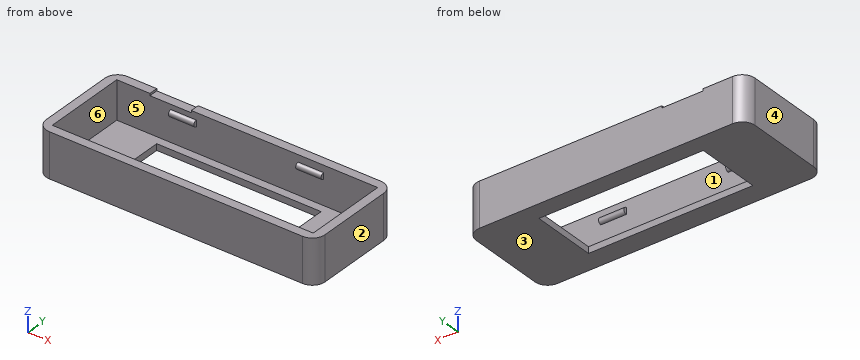
```python
from build123d import *

# Parameters (mm, degrees)
SKETCH010_W     = 43.8
SKETCH010_H     = 16.05
SKETCH010_W_2   = 41
SKETCH010_H_2   = 13.25
PAD004_DEPTH    = 6
SKETCH011_W     = 43.8
SKETCH011_H     = 16.05
SKETCH011_W_2   = 25.832
SKETCH011_H_2   = 10.205235
PAD005_DEPTH    = 1
FILLET_R        = 2
SKETCH012_W     = 6.5
SKETCH012_H     = 4.714983
POCKET004_DEPTH = 8.026
SKETCH027_R     = 0.5
PAD006_DEPTH    = 2


with BuildPart() as part:
    # Sketch010 → Pad004 (new body)
    with BuildSketch(Plane.XY):
        Rectangle(SKETCH010_W, SKETCH010_H)
        Rectangle(SKETCH010_W_2, SKETCH010_H_2, mode=Mode.SUBTRACT)
    extrude(amount=PAD004_DEPTH)

    # Sketch011 → Pad005 (join)
    with BuildSketch(Plane.XY):
        Rectangle(SKETCH011_W, SKETCH011_H)
        with Locations((-0.318418, 0.23483)):
            Rectangle(SKETCH011_W_2, SKETCH011_H_2, mode=Mode.SUBTRACT)
    extrude(amount=-PAD005_DEPTH)

    # Fillet
    fillet_edges = [part.edges().sort_by_distance(p)[0] for p in [
        (-21.9, -8.025, 3),
        (21.9, -8.025, 3),
        (-21.9, 8.025, 3),
        (21.9, 8.025, 3),
    ]]
    fillet(fillet_edges, radius=FILLET_R)

    # Sketch012 → Pocket004 (cut, through all)
    with BuildSketch(Plane.XZ):
        with Locations((-12.036756, 8.023509)):
            Rectangle(SKETCH012_W, SKETCH012_H)
    extrude(amount=-POCKET004_DEPTH, mode=Mode.SUBTRACT)

    # Sketch027 → Pad006 (join, symmetric)
    with BuildSketch(Plane.YZ.offset(10)):
        with Locations((6.62, 4.4)):
            Circle(SKETCH027_R)
        with Locations((-6.62, 4.4)):
            Circle(SKETCH027_R)
    pad006 = extrude(amount=PAD006_DEPTH, both=True)

    # Mirrored001: Pad006 across YZ
    add(pad006.mirror(Plane.YZ))


solid = part.part
```
Model file for the job. Use its own axes, mm. Face numbers are marked on the shaded views. A direction names the side the tool comes from. Give positions to 0.01 mm unless a question says otherwise; leave off trailing zeros. Loops run counter-clockwise (first coordinate to the right, second up) from the corner with the lowest first, then second, coordinate; pieces in that order, holes last. Notation, with made-up numbers: (-27, -2.5) - (19, -2.5) arc R22 cw to (19, 35.5) - close; hole circle Ø3 at (61.25, 59.25). An arc over 180 degrees is marked (long way). One line per item, written item: value. Start each with the question number.
1. Slice it at B-B (y = 2). List the corners of the cut face in (x, z), plus the area to 3 significant figures.
2. Which spindle directions (+Z, -Z, +X, -X, +Y, -Y) get a long thin tool onto all of the face, cutting with end or side? Do the marked faces 4, 5 and 6. Say none if no direction does.
3. Probe L1, parallel to X at y = 6, z = 5.75; L2, parallel to Y at x = -5, z = 1.75 (3 decimals); L3, parallel to Z at x = -14, y = 4.25. List the from-to ranges inside material, lowest first. Write a range as from..to.
4. Pull direction Z, two halves, no side cores. Call the marked faces 1, 2 and 3: pulls with the +Z half, pulls with the -Z half, needs draft (parallel to the pull), parting line crosses it, or undercut.
5. Slice it at A-A (x = -4.5). List the corners of the cut face in (y, z) (3 decimals).
6. Pin check, flat tips, straight feed: pin 1 (0.6 mm diameter, centred on y = -6.5, z = 4.5, fed in from -X); pin 2 (2 mm diameter, centred on x = -7, y = -4, fed in from +Z); pin 3 (0.7 mm diameter, centred on x = -11.5, y = 7.5, fed in from +Z). Stop position of each tip, or through.
7. Slice it at C-C (z = 4.4). List the corners of the cut face in (x, y) (3 decimals).
8. Slice it at D-D (y = -5.5). List the corners of the cut face in (x, z).
Solution:
1. outline: (-21.9, -1) - (-13.23, -1) - (-13.23, 0) - (-20.5, 0) - (-20.5, 6) - (-21.9, 6) - close; (12.6, -1) - (21.9, -1) - (21.9, 6) - (20.5, 6) - (20.5, 0) - (12.6, 0) - close
1. area: 34.8 mm^2
2. face 4: +Z, -Z, -X, +Y, -Y
2. face 5: none
2. face 6: +Z
3. L1: x = -21.9..-20.5, 20.5..21.9
3. L2: y = -8.025..-6.625, 6.625..8.025
3. L3: z = -1..0
4. face 1: undercut
4. face 2: needs draft
4. face 3: pulls with the -Z half
5. outline: (-8.025, -1) - (-4.868, -1) - (-4.868, 0) - (-6.625, 0) - (-6.625, 6) - (-8.025, 6) - close; (5.337, -1) - (8.025, -1) - (8.025, 6) - (6.625, 6) - (6.625, 0) - (5.337, 0) - close
6. pin 1: stops at x = -21.89
6. pin 2: stops at z = 0
6. pin 3: stops at z = 5.67
7. outline: (-21.9, -6.025) arc R2 ccw to (-19.9, -8.025) - (19.9, -8.025) arc R2 ccw to (21.9, -6.025) - (21.9, 6.025) arc R2 ccw to (19.9, 8.025) - (-19.9, 8.025) arc R2 ccw to (-21.9, 6.025) - close; hole (-20.5, -6.625) - (-12, -6.625) - (-12, -6.12) - (-8, -6.12) - (-8, -6.625) - (8, -6.625) - (8, -6.12) - (12, -6.12) - (12, -6.625) - (20.5, -6.625) - (20.5, 6.625) - (12, 6.625) - (12, 6.12) - (8, 6.12) - (8, 6.625) - (-8, 6.625) - (-8, 6.12) - (-12, 6.12) - (-12, 6.625) - (-20.5, 6.625) - close
8. outline: (-21.9, -1) - (21.9, -1) - (21.9, 6) - (20.5, 6) - (20.5, 0) - (-20.5, 0) - (-20.5, 6) - (-21.9, 6) - close
